Read the model definition and answer for the solid it produces. Units are mm, in the model's axes. A direction names the side the tool comes from. Round coordinates to 2 decimals unless told otherwise and drop trailing zeros. Order: outer loops, then holes, each group sorted by start corner. A loop starts at its lowest first (then second) coordinate and runs counter-clockwise, first axis right, second up. Notation, with made-up numbers: (-4, 28) - (42, 28) arc R18 ccw to (42, 40) - close; hole circle Ø10 at (-24.5, 2). An arc over 180 degrees is marked (long way). Put each result on its own line as item: value. Start each with the question number.
Q1. Section B-B on z = -125 is taken. Give the vertices of the cut face in (x, y) (3 decimals).
Q2. For a pull along X with two mould halves and no side action, classify faces 3 (the face through (165.097, 0.776, -108.534)), 4 (the face through (178.45, 0.78, -41.94)), 5 (the face through (134, 1.575, -82)) as pulls with the +X half, pulls with the -X half, needs draft (parallel to the pull), parting line crosses it, or undercut.
Q3. Which of the six approach directions +Z, -Z, +X, -X, +Y, -Y give full straight-line access (tool end or side, diameter ignored) to faces 1 (the face through (134, 0, -82)), 2 (the face through (179.24, 0.78, -174.75))?
Q4. Each of these flat-tipped pins is pushed along its axis until it touches: pin 1 Ø0.5 at (x, y) = (75, 1) entering from +Z (3 decimals); pin 2 Ø0.5 at (y, z) = (0.5, -100) entering from +X (3 decimals); pin 3 Ø0.5 at (y, z) = (1, -149) entering from -X (3 decimals). Where does it stop, or does it pass through?
Q5. Section A-A on x = 61 is taken. Give the vertices of the cut face in (y, z) (3 decimals), then the cut area to 3 significant figures.
Q6. Section C-C on z = -31 is taken. Give the vertices of the cut face in (x, y) (3 decimals), then the cut area to 3 significant figures.
Q7. Find the intervals of material crossed by line 1 along X through (y, z) = (0.6, -108.5) (3 decimals); line 2 along Z through (x, y) = (106, 1.15) (3 decimals); line 3 along Z through (x, y) = (110.5, 1.2) (3 decimals), in increasing order. Write a range as from..to.
Q8. Section D-D on z = -93 is taken. Give the vertices of the cut face in (x, y) (3 decimals).
from build123d import *

# Parameters (mm, degrees)
BOSS_EXTRUDE1_DEPTH = 1.5748


with BuildPart() as part:
    # Sketch1 → Boss-Extrude1 (new body)
    with BuildSketch(Plane(origin=(0, 0, 0), x_dir=(1, 0, 0), z_dir=(0, 1, 0))):
        with BuildLine():
            Line((219.075, 15.554259867), (219.075, 200.345740133))
            ThreePointArc((219.075, 200.345740133), (227.125320151, 227.125320151), (200.345740133, 219.075))
            Line((200.345740133, 219.075), (15.554259867, 219.075))
            ThreePointArc((15.554259867, 219.075), (-11.225320151, 227.125320151), (-3.175, 200.345740133))
            Line((-3.175, 200.345740133), (-3.175, 15.554259867))
            ThreePointArc((-3.175, 15.554259867), (-11.225320151, -11.225320151), (15.554259867, -3.175))
            Line((15.554259867, -3.175), (200.345740133, -3.175))
            ThreePointArc((200.345740133, -3.175), (227.125320151, -11.225320151), (219.075, 15.554259867))
        make_face()
        with BuildLine():
            Line((15.554259867, 3.175), (200.345740133, 3.175))
            ThreePointArc((200.345740133, 3.175), (201.233412421, 6.075099489), (202.656413342, 8.753458598))
            Line((202.656413342, 8.753458598), (146.053677431, 65.356194509))
            ThreePointArc((146.053677431, 65.356194509), (107.95, 50.8), (69.846322569, 65.356194509))
            Line((69.846322569, 65.356194509), (13.243586658, 8.753458598))
            ThreePointArc((13.243586658, 8.753458598), (14.666587579, 6.075099489), (15.554259867, 3.175))
        make_face(mode=Mode.SUBTRACT)
        with BuildLine():
            Line((8.753458598, 13.243586658), (65.356194509, 69.846322569))
            ThreePointArc((65.356194509, 69.846322569), (50.8, 107.95), (65.356194509, 146.053677431))
            Line((65.356194509, 146.053677431), (8.753458598, 202.656413342))
            ThreePointArc((8.753458598, 202.656413342), (6.075099489, 201.233412421), (3.175, 200.345740133))
            Line((3.175, 200.345740133), (3.175, 15.554259867))
            ThreePointArc((3.175, 15.554259867), (6.075099489, 14.666587579), (8.753458598, 13.243586658))
        make_face(mode=Mode.SUBTRACT)
        with BuildLine():
            Line((212.725, 15.554259867), (212.725, 200.345740133))
            ThreePointArc((212.725, 200.345740133), (209.824900511, 201.233412421), (207.146541402, 202.656413342))
            Line((207.146541402, 202.656413342), (150.543805491, 146.053677431))
            ThreePointArc((150.543805491, 146.053677431), (165.1, 107.95), (150.543805491, 69.846322569))
            Line((150.543805491, 69.846322569), (207.146541402, 13.243586658))
            ThreePointArc((207.146541402, 13.243586658), (209.824900511, 14.666587579), (212.725, 15.554259867))
        make_face(mode=Mode.SUBTRACT)
        with BuildLine():
            Line((15.554259867, 212.725), (200.345740133, 212.725))
            ThreePointArc((200.345740133, 212.725), (201.233412421, 209.824900511), (202.656413342, 207.146541402))
            Line((202.656413342, 207.146541402), (146.053677431, 150.543805491))
            ThreePointArc((146.053677431, 150.543805491), (107.95, 165.1), (69.846322569, 150.543805491))
            Line((69.846322569, 150.543805491), (13.243586658, 207.146541402))
            ThreePointArc((13.243586658, 207.146541402), (14.666587579, 209.824900511), (15.554259867, 212.725))
        make_face(mode=Mode.SUBTRACT)
    extrude(amount=BOSS_EXTRUDE1_DEPTH)


solid = part.part
Findings:
1. outline: (-3.175, 0) - (3.175, 0) - (3.175, 1.575) - (-3.175, 1.575) - close; (53.403, 0) - (162.497, 0) - (162.497, 1.575) - (53.403, 1.575) - close; (212.725, 0) - (219.075, 0) - (219.075, 1.575) - (212.725, 1.575) - close
2. face 3: undercut
2. face 4: undercut
2. face 5: needs draft
3. face 1: +Z, -Z, +X, -X, -Y
3. face 2: +Y, -Y
4. pin 1: z = 3.175
4. pin 2: x = 219.075
4. pin 3: x = -3.175
5. outline: (0, -219.075) - (1.575, -219.075) - (1.575, -212.725) - (0, -212.725) - close; (0, -159.39) - (1.575, -159.39) - (1.575, -150.41) - (0, -150.41) - close; (0, -140.536) - (1.575, -140.536) - (1.575, -75.364) - (0, -75.364) - close; (0, -65.49) - (1.575, -65.49) - (1.575, -56.51) - (0, -56.51) - close; (0, -3.175) - (1.575, -3.175) - (1.575, 3.175) - (0, 3.175) - close
5. area: 151 mm2
6. outline: (-3.175, 0) - (3.175, 0) - (3.175, 1.575) - (-3.175, 1.575) - close; (26.51, 0) - (35.49, 0) - (35.49, 1.575) - (26.51, 1.575) - close; (180.41, 0) - (189.39, 0) - (189.39, 1.575) - (180.41, 1.575) - close; (212.725, 0) - (219.075, 0) - (219.075, 1.575) - (212.725, 1.575) - close
6. area: 48.3 mm2
7. line 1: -3.175..3.175, 50.803..165.097, 212.725..219.075
7. line 2: -219.075..-212.725, -165.067..-50.833, -3.175..3.175
7. line 3: -219.075..-212.725, -165.043..-50.857, -3.175..3.175
8. outline: (-3.175, 0) - (3.175, 0) - (3.175, 1.575) - (-3.175, 1.575) - close; (52.79, 0) - (163.11, 0) - (163.11, 1.575) - (52.79, 1.575) - close; (212.725, 0) - (219.075, 0) - (219.075, 1.575) - (212.725, 1.575) - close
